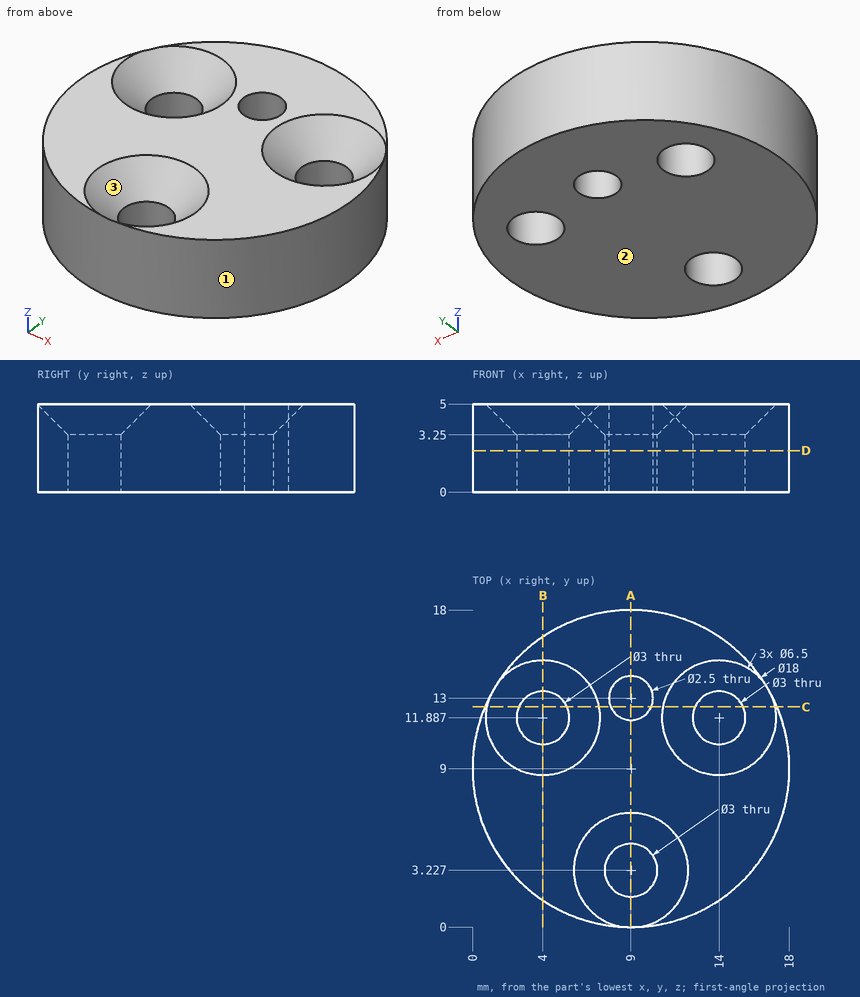
Job drawing, mm, ordinate dimensions from the low corner. One solid piece. Give positions to 0.01 mm unless a question says otherwise; leave off trailing zeros. Loops run counter-clockwise (first coordinate to the right, second up) from the corner with the lowest first, then second, coordinate; pieces in that order, holes last. Notation, with made-up numbers: (-8, -25) -> (-4, -25) arc R25 ccw to (-4, 10) -> close; hole circle Ø8 at (19.5, -13.75). An arc over 180 degrees is marked (long way). Write each question's results on one line, items separated by ' | '. Start each with the question number.
Q1. Pull direction Y, two halves, no side cores. Call the marked faces 1, 2 and 3: +Y half, -Y half, draft (parallel to the pull), parting line (faces both ways), or undercut.
Q2. Wall check: L1, parallel to Y at x = 9, z = 1.2; L2, parallel to Y at x = 9.75, z = 3.9; L3, parallel to X at y = 9.25, z = 1.45. Give the ranges that are in metal, low to high.
Q3. Band-saw the part on C-C on y = 12.5. Count the separate pieces of the cut face and the enclosed holes in it.
Q4. Band-saw the part on A-A on x = 9. List the corners of the cut face in (y, z).
Q5. Band-saw the part on D-D on z = 2.35. List the corners of the cut face in (x, y), plus the area to 3 significant figures.
Q6. Pin check, flat tips, straight feed: P1, Ø1.5, axis at x = 10, z = 1, coming from the -Y side; P2, Ø2.5, axis at x = 4, y = 11.89, coming from the +Z side; P3, Ø4, axis at x = 9, y = 3.23, coming from the +Z side (1 decimal); P4, Ø1, axis at x = 6.5, z = 1, coming from the -Y side (1 decimal). Stop position of each tip, or through.
Q7. Band-saw the part on B-B on x = 4. List the corners of the cut face in (y, z).
Results are:
1) face 1: parting line | face 2: draft | face 3: undercut
2) L1: y = 0 to 1.73, 4.73 to 11.75, 14.25 to 18 | L2: y = 0.03 to 1.21, 5.24 to 12, 14 to 17.97 | L3: x = 0 to 18
3) separate pieces: 4 | enclosed holes: 0
4) outline: (0, 0) -> (1.73, 0) -> (1.73, 3.25) -> (0, 4.98) -> close; (4.73, 0) -> (11.75, 0) -> (11.75, 5) -> (6.48, 5) -> (4.73, 3.25) -> close; (14.25, 0) -> (18, 0) -> (18, 5) -> (14.25, 5) -> close
5) outline: circle Ø18 at (9, 9); hole circle Ø3 at (4, 11.89); hole circle Ø3 at (9, 3.23); hole circle Ø2.5 at (9, 13); hole circle Ø3 at (14, 11.89) | area: 228 mm²
6) P1: stops at y = 0 | P2: passes through | P3: stops at z = 3.8 | P4: stops at y = 0.2
7) outline: (1.52, 0) -> (10.39, 0) -> (10.39, 3.25) -> (8.64, 5) -> (1.52, 5) -> close; (13.39, 0) -> (16.48, 0) -> (16.48, 5) -> (15.14, 5) -> (13.39, 3.25) -> close
